Geometry check sheet. Reference: the model listing, model coordinates, mm. A direction names the side the tool comes from. Coordinates: 2 decimals unless noted, no trailing zeros. Write each loop counter-clockwise with the first axis right and the second up, starting at its lowest first coordinate (ties: lowest second). Pieces come first, ordered by that corner, then holes. Notation, with made-up numbers: (11, -28.75) -> (69, -28.75) arc R11 cw to (69, -24.75) -> close; hole circle Ø8 at (54, -14). An arc over 180 degrees is marked (long way). One line per question, with ' | ' between items.
from build123d import *

# Parameters (mm, degrees)
BOSS_EXTRUDE1_DEPTH = 40
SKETCH3_R           = 15
BOSS_EXTRUDE2_DEPTH = 10
BOSS_EXTRUDE3_START = 10
SKETCH4_R           = 15
BOSS_EXTRUDE3_DEPTH = 10
SKETCH5_W           = 60
SKETCH5_H           = 25
CUT_EXTRUDE1_DEPTH  = 203.25937939
SKETCH6_R           = 15
CUT_EXTRUDE2_DEPTH  = 198.569877641


with BuildPart() as part:
    # Sketch1 → Boss-Extrude1 (new body)
    with BuildSketch(Plane.XY):
        with BuildLine():
            Line((-55.503676682, 25), (164.496323318, 25))
            ThreePointArc((164.496323318, 25), (189.496323318, 0), (164.496323318, -25))
            Line((164.496323318, -25), (-55.503676682, -25))
            ThreePointArc((-55.503676682, -25), (-80.503676682, 0), (-55.503676682, 25))
        make_face()
    extrude(amount=BOSS_EXTRUDE1_DEPTH)

    # Sketch3 → Boss-Extrude2 (add)
    with BuildSketch(Plane.XY.offset(40)):
        with Locations((-55.503676682, 0)):
            Circle(SKETCH3_R)
    extrude(amount=BOSS_EXTRUDE2_DEPTH)

    # Sketch4 → Boss-Extrude3 (add)
    with BuildSketch(Plane(origin=(0, 0, 0), x_dir=(-1, 0, 0), z_dir=(0, 0, -1)).offset(BOSS_EXTRUDE3_START)):
        with Locations(Location((55.503676682, 0, 0), (0, 0, 180))):
            Circle(SKETCH4_R)
    extrude(amount=-BOSS_EXTRUDE3_DEPTH)

    # Sketch5 → Cut-Extrude1 (cut, through all)
    with BuildSketch(Plane(origin=(0, 25, 0), x_dir=(1, 0, 0), z_dir=(0, 1, 0))):
        with Locations((159.496323318, -20)):
            Rectangle(SKETCH5_W, SKETCH5_H)
    extrude(amount=-CUT_EXTRUDE1_DEPTH, mode=Mode.SUBTRACT)

    # Sketch6 → Cut-Extrude2 (cut, through all)
    with BuildSketch(Plane.XY.offset(40)):
        with Locations((164.496323318, 0)):
            Circle(SKETCH6_R)
    extrude(amount=-CUT_EXTRUDE2_DEPTH, mode=Mode.SUBTRACT)


solid = part.part
1. Cross-section at B-B on y = -19. Record the boundary of the cut face in (x, z), and give its area (3 significant figures).
Worked answers:
outline: (-71.75, 0) -> (180.74, 0) -> (180.74, 7.5) -> (129.5, 7.5) -> (129.5, 32.5) -> (180.74, 32.5) -> (180.74, 40) -> (-71.75, 40) -> close | area: 8,820 mm²
2. Cross-section at D-D on z = 19.5. Record the boundary of the cut face in (x, y), and give its area (3 significant figures).
Worked answers:
outline: (-55.5, -25) -> (129.5, -25) -> (129.5, 25) -> (-55.5, 25) arc R25 ccw to start | area: 10,200 mm²
3. Cross-section at C-C on x = -15. Record the boundary of the cut face in (y, z), and give its area (3 significant figures).
Worked answers:
outline: (-25, 0) -> (25, 0) -> (25, 40) -> (-25, 40) -> close | area: 2,000 mm²
4. Mould release check, pull along Z, two halves, no side actions. Record for faces 1 (the face through (146, 0, 32.5)), 2 (the face through (56, -25, 20)), 3 (the face through (129.496, 0, 20)), 4 (the face through (56, 0, 0)): released by +Z, released by -Z, zero draft, split by the parting line, or undercut.
Worked answers:
face 1: undercut | face 2: zero draft | face 3: undercut | face 4: released by -Z
5. Cross-section at A-A on y = 0. Record the boundary of the cut face in (x, z), and give its area (3 significant figures).
Worked answers:
outline: (-80.5, 0) -> (-70.5, 0) -> (-70.5, -10) -> (-40.5, -10) -> (-40.5, 0) -> (149.5, 0) -> (149.5, 7.5) -> (129.5, 7.5) -> (129.5, 32.5) -> (149.5, 32.5) -> (149.5, 40) -> (-40.5, 40) -> (-40.5, 50) -> (-70.5, 50) -> (-70.5, 40) -> (-80.5, 40) -> close; (179.5, 0) -> (189.5, 0) -> (189.5, 7.5) -> (179.5, 7.5) -> close; (179.5, 32.5) -> (189.5, 32.5) -> (189.5, 40) -> (179.5, 40) -> close | area: 9,450 mm²
6. Material ranges on line 1 (Z direction, x = 154, y = 15.5); line 2 (Z direction, x = -1.5, y = 6); line 3 (X direction, y = -0.5, z = 17), recorded low to high. Write a range as from..to.
Worked answers:
line 1: 0..7.5, 32.5..40 | line 2: 0..40 | line 3: -80.5..129.5
7. Go/stop test with flat-tipped pins: P1, Ø1.5, axis at y = -18.5, z = 12.5, coming from the -X side; P2, Ø20, axis at y = -3.5, z = 20, coming from the +X side; P3, Ø15, axis at x = 58, y = 6.5, coming from the -Z side; P4, Ø24, axis at x = 164.5, y = 0, coming from the -Z side. Record where each tip stops, or that it passes through.
Worked answers:
P1: x = -73.11 | P2: x = 129.5 | P3: z = 0 | P4: through
8. Tool access check on faces 5 (the face through (-70.49, 0.66, 44.93)), 6 (the face through (146, 0, 7.5)), 7 (the face through (-70.49, -0.66, -5.07)), 8 (the face through (-56, 0, -10)). Record the directions out of +Z, -Z, +X, -X, +Y, -Y that give a thin tool (end or side, any length) a straight path to the whole face; none if there is none.
Worked answers:
face 5: +Z | face 6: +X, +Y, -Y | face 7: -Z | face 8: -Z, +X, -X, +Y, -Y
